Autodesk Inventor part; units mm, degrees
ref_plane "Work Plane1" through (0, 0, 23) normal (0, 0, 1) x (1, 0, 0)
ref_plane "Work Plane2" through (0, 0, 23) normal (0, 0, 1) x (1, 0, 0)
ref_plane "YZ Plane" through (0, 0, 0) normal (1, 0, 0) x (0, 1, 0)
sketch "Sketch1" plane through (0, 0, 0) normal (0, 0, 1) x (1, 0, 0)
  point P0 (0, 0)
sketch "Sketch2" plane through (0, 0, 0) normal (0, 0, 1) x (1, 0, 0)
  circle A0 centre (0, 0) radius 45
  circle A1 centre (0, 0) radius 66.5
  line L0 (-15, 42.4264) -> (-15, 50)
  line L1 (-15, 50) -> (15, 50)
  line L2 (15, 50) -> (15, 42.4264)
  line L3 (5, 88) -> (5, 87.8578)
  line L4 (0, 88) -> (0, 87.8578)
  line L5 (-5, 66.3118) -> (-2.5041, 87.9644)
  line L6 (5, 66.3118) -> (2.5, 88)
  arc A2 (2.5041, 87.9644) -> (-2.5041, 87.9644) centre (0, 0) ccw
  arc A3 (72.6365, 49.6783) -> (72.4155, 50) centre (0, 0) ccw
  arc A4 (84.4329, 24.8009) -> (82.8853, 29.564) centre (0, 0) ccw
  arc A5 (49.6783, -72.6365) -> (53.73, -69.6928) centre (0, 0) ccw
  arc A6 (-53.73, -69.6928) -> (-49.6783, -72.6365) centre (0, 0) ccw
  arc A7 (-82.8853, 29.564) -> (-84.4329, 24.8009) centre (0, 0) ccw
  line L7 (-31.5392, 58.5451) -> (-38.0659, 79.3409)
  line L8 (-22.4037, 62.6125) -> (-33.509, 81.4088)
  arc A8 (-33.4907, 81.378) -> (-38.0659, 79.3409) centre (0, 0) ccw
  line L9 (-52.6249, 40.6555) -> (-67.0458, 56.9987)
  line L10 (-45.9336, 48.087) -> (-63.7239, 60.7414)
  arc A9 (-63.6947, 60.7206) -> (-67.0458, 56.9987) centre (0, 0) ccw
  line L11 (-64.6113, 15.7362) -> (-84.4329, 24.8009)
  line L12 (-61.5211, 25.2467) -> (-82.9204, 29.5711)
  arc A10 (-82.8853, 29.564) -> (-84.4329, 24.8009) centre (0, 0) ccw
  line L13 (-65.4259, -11.9041) -> (-87.2207, -11.6852)
  line L14 (-66.4711, -1.9589) -> (-87.7792, -6.7122)
  arc A11 (-87.7442, -6.7044) -> (-87.2207, -11.6852) centre (0, 0) ccw
  line L15 (-54.9277, -37.486) -> (-74.9273, -46.1508)
  line L16 (-59.9277, -28.8258) -> (-77.4602, -41.8349)
  arc A12 (-77.4314, -41.8136) -> (-74.9273, -46.1508) centre (0, 0) ccw
  line L17 (-34.932, -56.5863) -> (-49.6783, -72.6365)
  line L18 (-43.0222, -50.7084) -> (-53.7476, -69.724)
  arc A13 (-53.73, -69.6928) -> (-49.6783, -72.6365) centre (0, 0) ccw
  line L19 (-8.8963, -65.9023) -> (-15.8394, -86.5628)
  line L20 (-18.6777, -63.8231) -> (-20.7416, -85.5572)
  arc A14 (-20.7382, -85.5215) -> (-15.8394, -86.5628) centre (0, 0) ccw
  line L21 (18.6777, -63.8231) -> (20.7382, -85.5215)
  line L22 (8.8963, -65.9023) -> (15.8509, -86.5968)
  arc A15 (15.8394, -86.5628) -> (20.7382, -85.5215) centre (0, 0) ccw
  line L23 (43.0222, -50.7084) -> (53.73, -69.6928)
  line L24 (34.932, -56.5863) -> (49.7026, -72.663)
  arc A16 (49.6783, -72.6365) -> (53.73, -69.6928) centre (0, 0) ccw
  line L25 (59.9277, -28.8258) -> (77.4314, -41.8136)
  line L26 (54.9277, -37.486) -> (74.9602, -46.1651)
  arc A17 (74.9273, -46.1508) -> (77.4314, -41.8136) centre (0, 0) ccw
  line L27 (66.4711, -1.9589) -> (87.7442, -6.7044)
  line L28 (65.4259, -11.9041) -> (87.2566, -11.6848)
  arc A18 (87.2207, -11.6852) -> (87.7442, -6.7044) centre (0, 0) ccw
  line L29 (61.5211, 25.2467) -> (82.8853, 29.564)
  line L30 (64.6113, 15.7362) -> (84.4655, 24.8159)
  arc A19 (84.4329, 24.8009) -> (82.8853, 29.564) centre (0, 0) ccw
  line L31 (45.9336, 48.087) -> (63.6947, 60.7206)
  line L32 (52.6249, 40.6555) -> (67.0696, 57.0256)
  arc A20 (67.0458, 56.9987) -> (63.6947, 60.7206) centre (0, 0) ccw
  line L33 (22.4037, 62.6125) -> (33.4907, 81.378)
  line L34 (31.5392, 58.5451) -> (38.0767, 79.3752)
  arc A21 (38.0659, 79.3409) -> (33.4907, 81.378) centre (0, 0) ccw
  point P0 (15, 46.2132)
  point P1 (-15, 46.2132)
  point P2 (5, 77.1559)
  point P3 (0, 77.1559)
  point P4 (0, -88)
  point P5 (-82.8853, 29.564)
  point P6 (-84.4329, 24.8009)
  point P7 (-53.73, -69.6928)
  point P8 (-49.6783, -72.6365)
  point P9 (49.6783, -72.6365)
  point P10 (53.73, -69.6928)
  point P11 (82.8853, 29.564)
  dimension "d2" = 90
  dimension "d3" = 21.5
  dimension "d4" = 30
  dimension "d5" = 50
  dimension "d6" = 88
  dimension "d7" = 15
  dimension "d10" = 38
  dimension "d17" = 360
extrude "Extrusion1" add sketch "Sketch2" along normal blind 46 contours A1
ref_plane "Work Plane1" through (0, 0, 23) normal (0, 0, 1) x (1, 0, 0)
ref_plane "Work Plane2" through (0, 0, 23) normal (0, 0, 1) x (1, 0, 0)
extrude "Extrusion2" add sketch "Sketch2" along normal blind 46 contours A1 L29 A4 L30 | L27 A18 L28 A1 | A1 L31 A20 L32 | L25 A17 L26 A1 | A1 L33 A21 L34 | L23 A5 L24 A1 | A1 L5 A2 L6 | L21 A15 L22 A1 | A1 L7 A8 L8 | L19 A14 L20 A1 | A1 L9 A9 L10 | L17 A6 L18 A1 | A1 L11 A7 L12 | L15 A12 L16 A1 | A1 L13 A11 L14
properties part number "Engranaje pequeño" material "Steel, Galvanized"
CAD build for the part. Positions are in the model's coordinates, mm. A direction names the side the tool comes from. Round coordinates to 2 decimals unless told otherwise and drop trailing zeros. Loops run counter-clockwise (first coordinate to the right, second up) from the corner with the lowest first, then second, coordinate; pieces in that order, holes last.
(1) Which spindle directions (+Z, -Z, +X, -X, +Y, -Y) get a long thin tool onto all of the face, cutting with end or side? Do faces 4 (the flat face through (-15, 46, 23)), 5 (the flat face through (54.69, 54.315, 22.678)), 6 (the flat face through (-48.301, -60.068, 22.678)), 7 (the flat face through (48.301, -60.068, 22.678)), 8 (the flat face through (-12.32, -76.09, 22.68)). Say none if no direction does.
(2) Drop flat-ended pins along their axis: pin 1 (12 mm diameter, centred on x = 26.5, z = 22, fed in from -Y); pin 2 (4 mm diameter, centred on y = 44.5, z = 27, fed in from +X); pin 3 (8.5 mm diameter, centred on y = 46, z = 33.5, fed in from -X). Give the stop position or say it passes through.
(3) Two-plate mould, pull along X, no slides. Class faces 1 (the cylindrical face through (83.68, 27.23, 22.68)), 2 (the cylindrical face through (-35.82, 80.38, 22.68)), 3 (the flat face through (-72.054, 27.375, 22.678)): +X half, -X half, draft (parallel to the pull), parting line (faces both ways), or undercut.
(4) Wall check: line 1 along Y through (x, z) = (0, 15.5); line 2 along X through (y, z) = (0, 29); line 3 along X through (y, z) = (77, 16). Give the ranges that are in metal, low to high.
(5) Cut at B-B (y = -14). Give the cut face in (x, z).
(6) Cut at A-A (x = 0). Give the cut face in (y, z).
Findings below:
1. face 4: +Z, -Z
1. face 5: +Z, -Z, +Y
1. face 6: +Z, -Z, -X
1. face 7: +Z, -Z, +X
1. face 8: +Z, -Z, -Y
2. pin 1: stops at y = -85.58
2. pin 2: stops at x = 57.78
2. pin 3: stops at x = -61.09
3. face 1: +X half
3. face 2: -X half
3. face 3: undercut
4. line 1: y = -66.5 to -45, 50 to 88
4. line 2: x = -66.5 to -45, 45 to 66.5
4. line 3: x = -37.33 to -30.9, -3.77 to 3.77, 30.9 to 37.33
5. outline: (-65.01, 0) - (-42.77, 0) - (-42.77, 46) - (-65.01, 46) - close; (42.77, 0) - (65.01, 0) - (65.01, 46) - (42.77, 46) - close
6. outline: (-66.5, 0) - (-45, 0) - (-45, 46) - (-66.5, 46) - close; (50, 0) - (88, 0) - (88, 46) - (50, 46) - close
